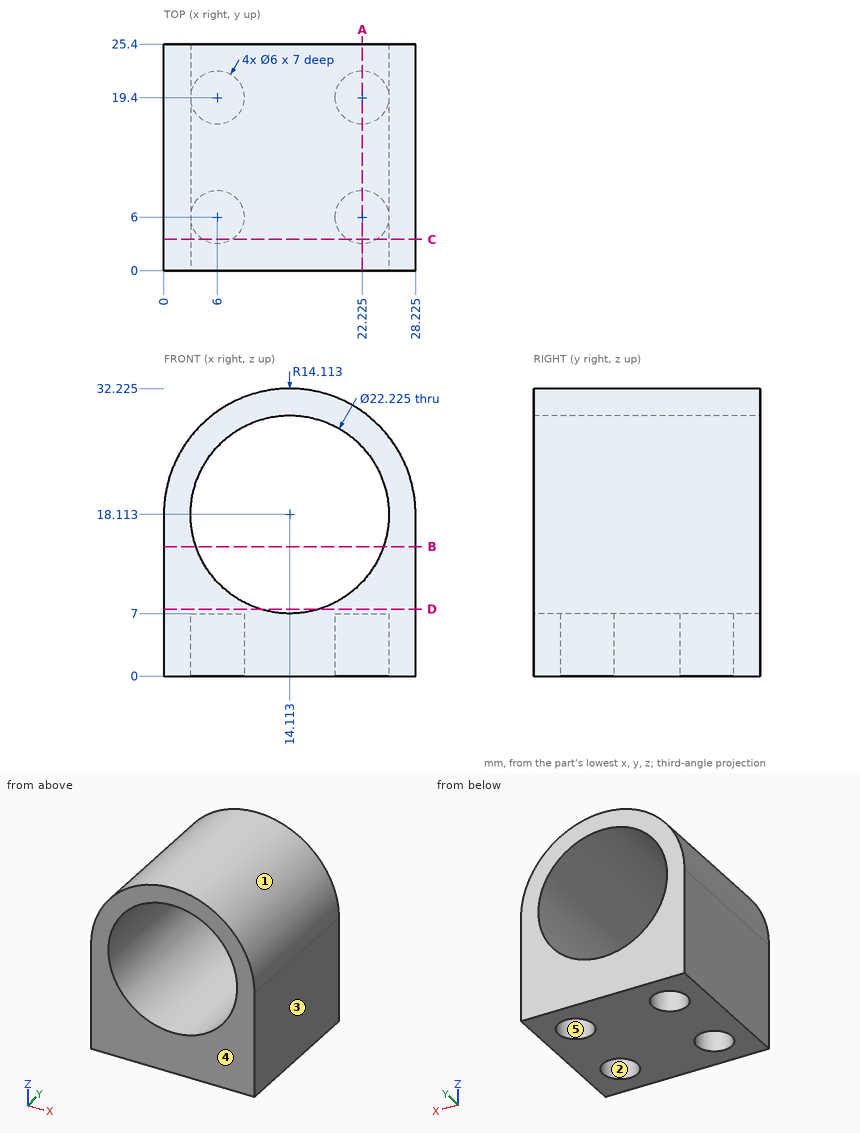
Geometry: see drawing. Coordinates: mm, zero at the bounding-box minimum. A direction names the side the tool comes from. Round coordinates to 2 decimals unless told otherwise and drop trailing zeros. Write each loop counter-clockwise with the first axis right and the second up, starting at its lowest first coordinate (ties: lowest second). Pieces come first, ordered by that corner, then holes.
Item 1: Section query C-C (y = 3.5). Return loops of the section in (x, z) (1 decimal).
Item 2: Section query D-D (z = 7.5). Return loops of the section in (x, y) (1 decimal).
Item 3: Pin query (flat end, axial travel): P1, Ø3, axis at x = 6, y = 20.5, coming from the -Z side; P2, Ø5, axis at x = 6, y = 19.4, coming from the +Z side; P3, Ø5.5, axis at x = 6, y = 6, coming from the +Z side. Return the tip coordinate at first contact, or that it passes through.
Item 4: Section query A-A (x = 22.25). Return loops of the section in (y, z) (1 decimal).
Item 5: Set-up query: the marked faces 1 and 2. Return all of +Z, -Z, +X, -X, +Y, -Y with unobstructed straight access to the full face (end or side cutting, diameter ignored); none if empty.
Item 6: Section query B-B (z = 14.5). Return loops of the section in (x, y) (1 decimal), plus the area to 3 significant figures.
Item 7: Mould query, pull axis Y, two halves, no side actions, for the marked faces 3, 4 and 5. Classes: +Y half, -Y half, draft (parallel to the pull), parting line (faces both ways), or undercut.
Item 8: Material intervals for L1, parallel to Y at x = 6, z = 3; L2, parallel to X at y = 20.5, z = 18 (1 decimal); L3, parallel to X at y = 8.25, z = 19.5, sorted ascending.
Completed:
1. outline: (0, 0) - (4.3, 0) - (4.3, 7) - (7.7, 7) - (7.7, 0) - (20.6, 0) - (20.6, 7) - (23.9, 7) - (23.9, 0) - (28.2, 0) - (28.2, 18.1) arc R14.1 ccw to (0, 18.1) - close; hole circle Ø22.2 at (14.1, 18.1)
2. outline: (0, 0) - (10.8, 0) - (10.8, 25.4) - (0, 25.4) - close; (17.4, 0) - (28.2, 0) - (28.2, 25.4) - (17.4, 25.4) - close
3. P1: stops at z = 7
3. P2: stops at z = 31.06
3. P3: stops at z = 31.17
4. outline: (0, 0) - (3, 0) - (3, 7) - (9, 7) - (9, 0) - (16.4, 0) - (16.4, 7) - (22.4, 7) - (22.4, 0) - (25.4, 0) - (25.4, 10.5) - (0, 10.5) - close; (0, 25.7) - (25.4, 25.7) - (25.4, 29.6) - (0, 29.6) - close
5. face 1: +Z, +Y, -Y
5. face 2: -Z
6. outline: (0, 0) - (3.6, 0) - (3.6, 25.4) - (0, 25.4) - close; (24.6, 0) - (28.2, 0) - (28.2, 25.4) - (24.6, 25.4) - close
6. area: 183 mm2
7. face 3: draft
7. face 4: -Y half
7. face 5: undercut
8. L1: y = 0 to 3, 9 to 16.4, 22.4 to 25.4
8. L2: x = 0 to 3, 25.2 to 28.2
8. L3: x = 0.07 to 3.09, 25.14 to 28.16
